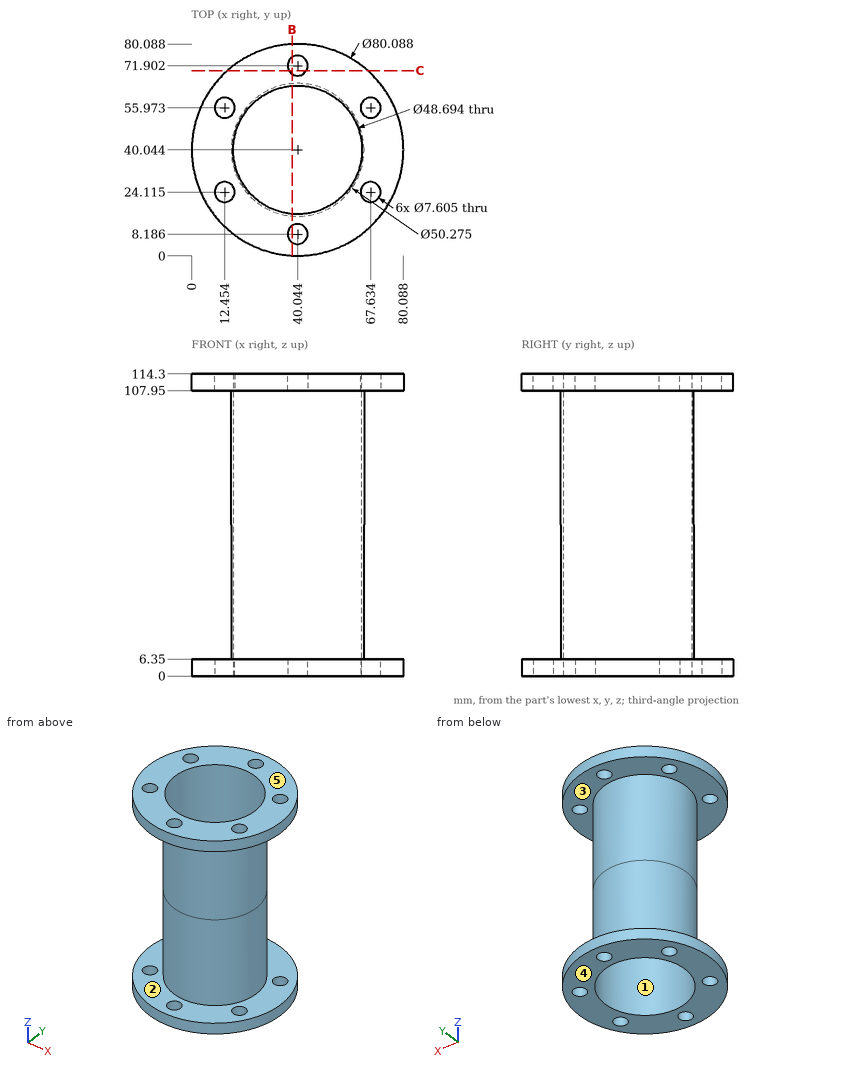
Study the drawing (mm; zero at the part's minimum x, y, z) and answer. A direction names the side the tool comes from. Round coordinates to 2 decimals unless told otherwise and drop trailing zeros. Write each loop counter-clockwise with the first axis right and the second up, starting at its lowest first coordinate (ties: lowest second). Pieces come first, ordered by that corner, then holes. Notation, with made-up numbers: (39, 87.25) - (72, 87.25) arc R21 cw to (72, 110.25) - close; hole circle Ø5 at (18, 7). An arc over 180 degrees is marked (long way). Return JSON: item names as keys, results as strings. Group by question number.
Q1. The mould has two halves that part along Z. Classify the marked faces 3, 4 and 5: released by +Z, released by -Z, zero draft, split by the parting line, or undercut.
Q2. The part is cut by section B-B on x = 38. Count the separate pieces of the cut face and the enclosed holes in it.
Q3. The part is cut by section C-C on y = 70. Write down the section's boundary in (x, z).
Q4. Find the intervals of material crossed by L1, parallel to Z at x = 6.5, y = 61; L2, parallel to Y at x = 40.5, z = 14.5; L3, parallel to Y at x = 25, z = 51.5 (1 decimal), in increasing order.
Q5. For the marked faces 1 and 2, determine the directions among +Z, -Z, +X, -X, +Y, -Y from which every point of the face is accessible in a straight line to the end or side of a thin tool.
Q6. Each of these flat-tipped pins is pushed along its axis until it touches: pin 1 Ø1 at (x, z) = (48, 18) entering from +Y; pin 2 Ø1.5 at (x, z) = (47, 33) entering from -Y (1 decimal); pin 3 Ø10 at (x, z) = (53.5, 101) entering from +Y. Where does it stop, or does it pass through?
Solved:
{
 "1": {"face 3": "undercut", "face 4": "released by -Z", "face 5": "released by +Z"},
 "2": {"separate pieces": "6", "enclosed holes": "0"},
 "3": {"outline": "(13.47, 0) - (36.75, 0) - (36.75, 6.35) - (13.47, 6.35) - close; (13.47, 107.95) - (36.75, 107.95) - (36.75, 114.3) - (13.47, 114.3) - close; (43.34, 0) - (66.62, 0) - (66.62, 6.35) - (43.34, 6.35) - close; (43.34, 107.95) - (66.62, 107.95) - (66.62, 114.3) - (43.34, 114.3) - close"},
 "4": {"L1": "0 to 6.35, 107.95 to 114.3", "L2": "14.91 to 15.7, 64.39 to 65.18", "L3": "19.9 to 20.9, 59.2 to 60.2"},
 "5": {"face 1": "+Z, -Z", "face 2": "none"},
 "6": {"pin 1": "y = 64.05", "pin 2": "y = 15.7", "pin 3": "y = 63.72"}
}
